Can you work these out from the model? Positions are in its coordinate system, mm. A direction names the side the tool comes from. Round coordinates to 2 decimals unless told otherwise and drop trailing zeros. Write each loop counter-clockwise with the first axis right and the second up, starting at its lowest first coordinate (ties: lowest second). Pieces come first, ordered by that corner, then holes. Notation, with made-up numbers: (-21.75, 10.25) - (-15.75, 10.25) arc R22 cw to (-15.75, 18.25) - close; hole circle Ø4 at (-8.5, 21.5). An arc over 180 degrees is marked (long way). One line per item, written item: value. Start each with the question number.
(1) I want a section at B-B on y = 7. List the corners of the cut face in (x, z) for me.
(2) On a 3-axis mill with a long thin cutter (end or side, diameter ignored), from which of +Z, -Z, +X, -X, +Y, -Y can I reach the whole of each face in a straight line? I mean faces 4 (the face through (0, 39.971, 22)), 5 (the face through (16.885, -18.046, 22.57)). Say none if no direction works.
(3) I want a section at D-D on x = 26. List the corners of the cut face in (y, z) for me.
(4) If I drill on L1, parallel to Y at x = -18, z = 20.5; L2, parallel to X at y = 16, z = 24; L3, parallel to X at y = -24, z = 24, over which ranges is the centre line in solid material (lowest first)? Write a range as from..to.
(5) I'm going to push flat-ended pins straight in: pin 1 Ø5 at (x, y) = (16.5, -18) entering from -Z; pin 2 Ø2 at (y, z) = (-28, 31) entering from +X; pin 3 Ø3 at (y, z) = (15, 16) entering from -X; pin 4 Ø2 at (y, z) = (-4.5, 36) entering from +X. Where does each tip first touch, or does it pass through?
(6) I want a section at A-A on z = 35. List the corners of the cut face in (x, y) for me, plus the area to 3 significant figures.
(7) Thinking about a two-plate mould opening in Z: for faces 1 (the face through (0, 1, 0)), 2 (the face through (16.87, 18.07, 22.57)), 3 (the face through (-18.59, -25.09, 22.18)), which applies, +Z half, -Z half, draft (parallel to the pull), parting line (faces both ways), or undercut?
(8) I want a section at C-C on z = 19. List the corners of the cut face in (x, y) for me, plus the area to 3 significant figures.
from build123d import *

# Parameters (mm, degrees)
BOSS_EXTRUDE1_DEPTH = 45
SKETCH3_R           = 5
CUT_EXTRUDE1_DEPTH  = 5
SKETCH4_R           = 5
CUT_EXTRUDE2_DEPTH  = 5
SKETCH5_R           = 5
CUT_EXTRUDE3_DEPTH  = 5
SKETCH6_R           = 5
CUT_EXTRUDE4_DEPTH  = 5


with BuildPart() as part:
    # Sketch2 → Boss-Extrude1 (new body)
    with BuildSketch(Plane.XY):
        Polygon((-10, 39.97114317), (10, 39.97114317), (32.5, 1), (32.5, -1), (10, -39.97114317), (-10, -39.97114317), (-32.5, -1), (-32.5, 1), align=None)
    extrude(amount=BOSS_EXTRUDE1_DEPTH)

    # Sketch3 → Cut-Extrude1 (cut)
    with BuildSketch(Plane(origin=(24.808012702, 14.322912811, 0), x_dir=(0, 0, -1), z_dir=(0.8660254037844365, 0.500000000000004, 0))):
        with Locations(Location((-22.5, 7.281943839, 0), (0, 0, 90))):
            Circle(SKETCH3_R)
    extrude(amount=-CUT_EXTRUDE1_DEPTH, mode=Mode.SUBTRACT)

    # Sketch4 → Cut-Extrude2 (cut)
    with BuildSketch(Plane(origin=(-24.808012702, 14.322912811, 0), x_dir=(0, 0, 1), z_dir=(-0.8660254037844253, 0.5000000000000234, 0))):
        with Locations(Location((22.5, 7.116025404, 0), (0, 0, 270))):
            Circle(SKETCH4_R)
    extrude(amount=-CUT_EXTRUDE2_DEPTH, mode=Mode.SUBTRACT)

    # Sketch5 → Cut-Extrude3 (cut)
    with BuildSketch(Plane(origin=(-24.808012702, -14.322912811, 0), x_dir=(0, 0, 1), z_dir=(-0.8660254037844344, -0.5000000000000075, 0))):
        with Locations(Location((22.5, -7.116025404, 0), (0, 0, 270))):
            Circle(SKETCH5_R)
    extrude(amount=-CUT_EXTRUDE3_DEPTH, mode=Mode.SUBTRACT)

    # Sketch6 → Cut-Extrude4 (cut)
    with BuildSketch(Plane(origin=(24.808012702, -14.322912811, 0), x_dir=(0, 0, -1), z_dir=(0.8660254037844365, -0.500000000000004, 0))):
        with Locations(Location((-22.5, -7.116025404, 0), (0, 0, 90))):
            Circle(SKETCH6_R)
    extrude(amount=-CUT_EXTRUDE4_DEPTH, mode=Mode.SUBTRACT)


solid = part.part
Established:
1. outline: (-29.04, 0) - (29.04, 0) - (29.04, 45) - (-29.04, 45) - close
2. face 4: +Z, -Z, +X, -X, +Y
2. face 5: none
3. outline: (-12.26, 0) - (12.26, 0) - (12.26, 45) - (-12.26, 45) - close
4. L1: -26.11..-23.9, -16.11..16.11, 23.9..26.11
4. L2: -23.84..-23.02, -18.07..18.07, 22.69..23.84
4. L3: -17.8..17.8
5. pin 1: z = 0
5. pin 2: x = 17.49
5. pin 3: x = -25.28
5. pin 4: x = 31.06
6. outline: (-32.5, -1) - (-10, -39.97) - (10, -39.97) - (32.5, -1) - (32.5, 1) - (10, 39.97) - (-10, 39.97) - (-32.5, 1) - close
6. area: 3,440 mm2
7. face 1: -Z half
7. face 2: undercut
7. face 3: draft
8. outline: (-32.5, -1) - (-23.04, -17.39) - (-18.71, -14.89) - (-15.13, -21.08) - (-19.46, -23.58) - (-10, -39.97) - (10, -39.97) - (19.46, -23.58) - (15.13, -21.08) - (18.71, -14.89) - (23.04, -17.39) - (32.5, -1) - (32.5, 1) - (22.95, 17.54) - (18.62, 15.04) - (15.05, 21.22) - (19.38, 23.72) - (10, 39.97) - (-10, 39.97) - (-19.46, 23.58) - (-15.13, 21.08) - (-18.71, 14.89) - (-23.04, 17.39) - (-32.5, 1) - close
8. area: 3,300 mm2
